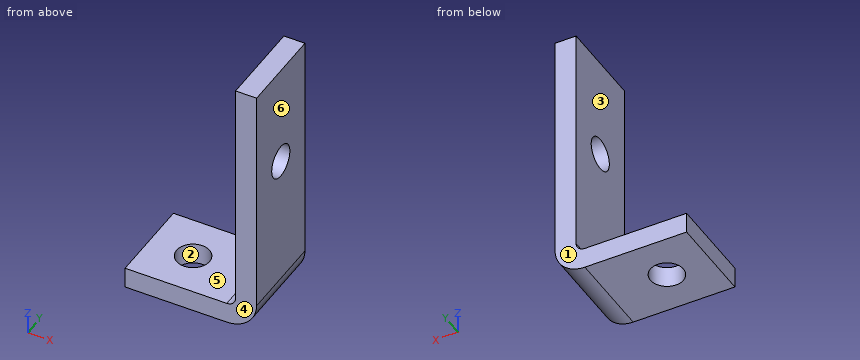
Autodesk Inventor part; units mm, degrees
ref_plane "YZ Plane" through (0, 0, 0) normal (1, 0, 0) x (0, 1, 0)
ref_plane "XZ Plane" through (0, 0, 0) normal (0, 1, 0) x (-1, 0, 0)
ref_plane "XY Plane" through (0, 0, 0) normal (0, 0, 1) x (1, 0, 0)
sketch "Sketch1" plane through (0, 0, 0) normal (0, 0, 1) x (1, 0, 0)
  circle A0 centre (0, 0) radius 2.3876
  line L0 (12.7, 0) -> (12.7, 6.35)
  line L1 (12.7, -6.35) -> (12.7, 0)
  line L2 (-6.35, -6.35) -> (-6.35, 6.35)
  line L3 (-6.35, 6.35) -> (12.7, 6.35)
  line L4 (-6.35, -6.35) -> (12.7, -6.35)
  dimension "d0" = 4.7752
  dimension "d1" = 6.35
  dimension "d4" = 12.7
  dimension "d22" = 19.05
  dimension "d23" = 12.7
extrude "Plate1" add sketch "Sketch1" along normal blind 3.048
sketch "Sketch2" plane through (9.652, 6.35, 0) normal (1, 0, 0) x (0, 1, 0)
  line L0 (-12.7, 0) -> (0, 0)
  line L1 (0, 0) -> (0, 38.1)
  line L2 (0, 38.1) -> (-12.7, 38.1)
  line L3 (-12.7, 38.1) -> (-12.7, 0)
edge flange "Flange1" height 38.1 angle 90 thickness 3.048 bend radius 1.27 thickness toward (1, 0, 0) relief tear relief width 3.048 relief depth 1.524 edges at (12.7, 3.175, 3.048) wall of the first edge with corners at (9.652, -6.35, 0) (9.652, 6.35, 0) (9.652, 6.35, 38.1) (9.652, -6.35, 38.1)
bend "Bend1"
corner "Corner1"
sketch "Sketch3" plane through (12.7, -6.35, 38.1) normal (1, 0, 0) x (0, 0, -1)
  circle A0 centre (14.732, 6.35) radius 2.3812
  line L0 (33.782, 0) -> (33.782, 12.7)
  line L1 (33.782, 0) -> (0, 0)
  point P0 (38.1, 6.35)
  dimension "d17" = 4.7625
  dimension "d20" = 6.35
  dimension "d21" = 19.05
extrude "Extrusion1" cut sketch "Sketch3" against normal blind 25.4
equation "\"d7\" = BendReliefWidth"
equation "\"d8\" = BendReliefDepth"
equation "\"d9\" = MinimumRemnant"
equation "\"d10\" = BendRadius"
equation "\"d14\" = CornerReliefSize"
equation "\"d15\" = GapSize"
equation "\"d16\" = JacobiRadiusSize"
equation "\"BendRadius\" = Thickness"
equation "\"BendReliefWidth\" = Thickness"
equation "\"BendReliefDepth\" = 0.5 * Thickness"
equation "\"CornerReliefSize\" = 4 * Thickness"
equation "\"MinimumRemnant\" = 2 * Thickness"
equation "\"TransitionRadius\" = BendRadius"
equation "\"JacobiRadiusSize\" = BendRadius"
equation "\"GapSize\" = Thickness"
equation "\"d6\" = BendRadius"
properties part number "PistonFrontHinge"
For this review, take the finished solid that the model builds, in its own axes (mm). Face numbers are marked on the shaded views. A direction names the side the tool comes from. Round coordinates to 2 decimals unless told otherwise and drop trailing zeros. Write each loop counter-clockwise with the first axis right and the second up, starting at its lowest first coordinate (ties: lowest second). Pieces come first, ordered by that corner, then holes. Notation, with made-up numbers: (88.25, 10) - (142.25, 10) arc R9 cw to (142.25, 20) - close; hole circle Ø7 at (8.25, 40.5). An arc over 180 degrees is marked (long way). Write item = value, one per line. Start each with the question number.
1. Consider section A-A on x = 0. State the section outline as (y, z) points, plus the area to 3 significant figures.
2. Draft analysis for pull direction Y (two halves, no side actions). For the marked faces 1, 2, 3 and 4, state which applies: released by +Y, released by -Y, zero draft, split by the parting line, or undercut.
3. Consider section D-D on y = -5.25. State the section outline as (x, z) points, plus the area to 3 significant figures.
4. Consider section C-C on z = 22.5. State the section outline as (x, y) points.
5. Wall thickness on L1, parallel to Y at x = 0, z = 0.9; L2, parallel to Z at x = 7.25, y = -5; L3, parallel to X at y = 5.75, z = 24: over which ranges is each line inside the solid? List them lowest first.
6. For the marked faces 5 and 6, list the 3-axis set-ups (+Z, -Z, +X, -X, +Y, -Y) from which the entire face can be reached by the end or side of a thin tool; tool diameter is ignored.
7. For pin 1 Ø5.5 at (x, y) = (0, 0) entering from +Z; pin 2 Ø6 at (y, z) = (0, 23.368) entering from -X, all flat-tipped, find the tip position at first contact; note any pin that passes through.
8. Consider section B-B on y = 0. State the section outline as (x, z) points, plus the area to 3 significant figures.
Evaluation:
q1.outline = (-6.35, 0) - (-2.39, 0) - (-2.39, 3.05) - (-6.35, 3.05) - close; (2.39, 0) - (6.35, 0) - (6.35, 3.05) - (2.39, 3.05) - close
q1.area = 24.2 mm2
q2.face_1 = released by +Y
q2.face_2 = undercut
q2.face_3 = zero draft
q2.face_4 = released by -Y
q3.outline = (-6.35, 0) - (8.38, 0) arc R4.32 ccw to (12.7, 4.32) - (12.7, 38.1) - (9.65, 38.1) - (9.65, 4.32) arc R1.27 cw to (8.38, 3.05) - (-6.35, 3.05) - close
q3.area = 161 mm2
q4.outline = (9.65, -6.35) - (12.7, -6.35) - (12.7, -2.22) - (9.65, -2.22) - close; (9.65, 2.22) - (12.7, 2.22) - (12.7, 6.35) - (9.65, 6.35) - close
q5.L1 = -6.35 to -2.39, 2.39 to 6.35
q5.L2 = 0 to 3.05
q5.L3 = 9.65 to 12.7
q6.face_5 = +Z, -X, +Y, -Y
q6.face_6 = +Z, -Z, +X, +Y, -Y
q7.pin_1 = 3.05
q7.pin_2 = 9.65
q8.outline = (-6.35, 0) - (-2.39, 0) - (-2.39, 3.05) - (-6.35, 3.05) - close; (2.39, 0) - (8.38, 0) arc R4.32 ccw to (12.7, 4.32) - (12.7, 20.99) - (9.65, 20.99) - (9.65, 4.32) arc R1.27 cw to (8.38, 3.05) - (2.39, 3.05) - close; (9.65, 25.75) - (12.7, 25.75) - (12.7, 38.1) - (9.65, 38.1) - close
q8.area = 132 mm2
